The listing builds one solid part. Answer for the finished solid, in the listing's coordinates (mm). A direction names the side the tool comes from. Give positions to 0.01 mm unless a question says otherwise; leave off trailing zeros. Loops run counter-clockwise (first coordinate to the right, second up) from the corner with the lowest first, then second, coordinate; pieces in that order, holes last. Notation, with made-up numbers: M 66,70.25 L 95,70.25 A12 cw 95,74.25 Z; hole C -23.75,28 d10. An arc over 180 degrees is marked long. One line per item, written item: value. Start each with the question number.
Q1. The mould has two halves that part along X. Classify faces 3 (the cylindrical face through (-26.78, -38.63, -18.9)), 4 (the flat face through (-38.1, -38, 0)), 5 (the flat face through (-1, 0, 0)): +X half, -X half, draft (parallel to the pull), parting line (faces both ways), or undercut.
Q2. A cutting plane is placed at B-B, the plane y = -15. Determine the outline of the cut face in (x, z).
Q3. A cutting plane is placed at A-A, the plane x = 25.4. Determine the outline of the cut face in (y, z).
Q4. Consider L1, parallel to Z at x = -25.4, y = -24; L2, parallel to Z at x = -28, y = -46.5; L3, parallel to X at y = -20.5, z = 13.5. Determine where each line is inside the solid, lowest interval first.
Q5. A flat-ended cylindrical pin translates along its axis: pin 1 (8 mm diameter, centred on x = -20, z = 10.5, fed in from -Y). Find the tip coordinate at first contact, or state that the pin passes through.
Q6. A cutting plane is placed at C-C, the plane z = 0. Determine the outline of the cut face in (x, y), and give its area (3 significant figures).
Q7. For faces 1 (the flat face through (0, -101.6, 0)), 2 (the flat face through (8, -76.2, 12)), determine the directions among +Z, -Z, +X, -X, +Y, -Y from which every point of the face is accessible in a straight line to the end or side of a thin tool.
Q8. A cutting plane is placed at D-D, the plane z = 14. Determine the outline of the cut face in (x, y).
from build123d import *

# Parameters (mm, degrees)
F0_W     = 76.2
F0_H     = 50.8
F1_DEPTH = 76.2
F2_R     = 6.35
F3_DEPTH = 76.201
F4_W     = 12.7
F4_H     = 25.4


with BuildPart() as f1:
    # F0 (on Front) → F1 (new body)
    with BuildSketch(Plane.XZ):
        Rectangle(F0_W, F0_H)
    extrude(amount=F1_DEPTH)

    # F2 (on face) → F3 (cut, through all)
    with BuildSketch(Plane.XZ.offset(76.2)):
        with Locations((-25.4, 12.7)):
            Circle(F2_R)
        with Locations((-25.4, -12.7)):
            Circle(F2_R)
        with Locations((25.4, 12.7)):
            Circle(F2_R)
        with Locations((25.4, -12.7)):
            Circle(F2_R)
    extrude(amount=-F3_DEPTH, mode=Mode.SUBTRACT)

    # F4 (on Top) → F5 (revolve)
    with BuildSketch(Plane.XY):
        with Locations((-6.35, -88.9)):
            Rectangle(F4_W, F4_H)
    revolve(axis=Axis((0, -88.9, 0), (0, -1, 0)))


solid = f1.part
Answer block:
1. face 3: undercut
1. face 4: -X half
1. face 5: draft
2. outline: M -38.1,-25.4 L 38.1,-25.4 L 38.1,25.4 L -38.1,25.4 Z; hole C -25.4,-12.7 d12.7; hole C -25.4,12.7 d12.7; hole C 25.4,-12.7 d12.7; hole C 25.4,12.7 d12.7
3. outline: M -76.2,-25.4 L 0,-25.4 L 0,-19.05 L -76.2,-19.05 Z; M -76.2,-6.35 L 0,-6.35 L 0,6.35 L -76.2,6.35 Z; M -76.2,19.05 L 0,19.05 L 0,25.4 L -76.2,25.4 Z
4. L1: -25.4 to -19.05, -6.35 to 6.35, 19.05 to 25.4
4. L2: -25.4 to -18.49, -6.91 to 6.91, 18.49 to 25.4
4. L3: -38.1 to -31.7, -19.1 to 19.1, 31.7 to 38.1
5. pin 1: y = -76.2
6. outline: M -38.1,-76.2 L -12.7,-76.2 L -12.7,-101.6 L 12.7,-101.6 L 12.7,-76.2 L 38.1,-76.2 L 38.1,0 L -38.1,0 Z
6. area: 6,450 mm^2
7. face 1: +Z, -Z, +X, -X, -Y
7. face 2: -Y
8. outline: M -38.1,-76.2 L -31.62,-76.2 L -31.62,0 L -38.1,0 Z; M -19.18,-76.2 L 19.18,-76.2 L 19.18,0 L -19.18,0 Z; M 31.62,-76.2 L 38.1,-76.2 L 38.1,0 L 31.62,0 Z
